```python
from build123d import *

# Parameters (mm, degrees)
F0_W     = 10
F0_H     = 20
F0_R     = 2.65
F1_DEPTH = 2.2
F2_R     = 0.5


with BuildPart() as f1:
    # F0 (on Top) → F1 (new body)
    with BuildSketch(Plane.XY):
        Rectangle(F0_W, F0_H)
        Circle(F0_R, mode=Mode.SUBTRACT)
    extrude(amount=F1_DEPTH)

    # F2
    f2_edges = [f1.edges().sort_by_distance(p)[0] for p in [
        (-2.65, 0, 2.2),
        (5, 0, 2.2),
        (0, 10, 2.2),
        (0, -10, 2.2),
        (-5, 0, 2.2),
    ]]
    fillet(f2_edges, radius=F2_R)


solid = f1.part
```
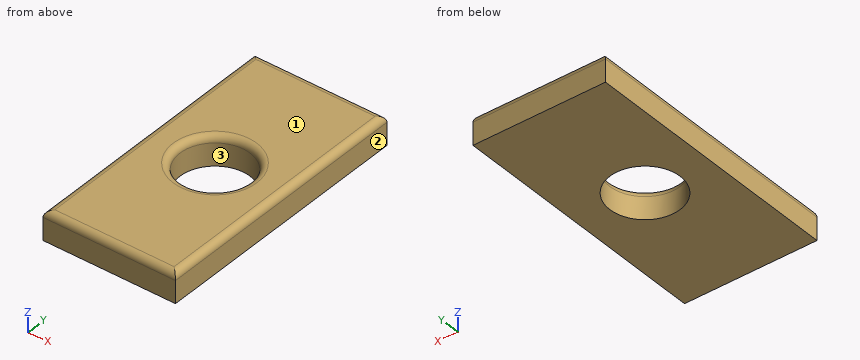
For this review, take the finished solid that the model builds, in its own axes (mm). Face numbers are marked on the shaded views. Coordinates: 2 decimals unless noted, no trailing zeros. Write each loop counter-clockwise with the first axis right and the second up, starting at its lowest first coordinate (ties: lowest second). Pieces come first, ordered by that corner, then holes. Notation, with made-up numbers: (3, -25.75) - (20, -25.75) arc R9 ccw to (20, -21.75) - close; hole circle Ø5 at (-26.75, -40). An arc over 180 degrees is marked (long way). Answer in a Markdown table with one row per item. Add a question column.
Q1. For probe 1 along Y at (x, z) = (0, 0.65); probe 2 along X at (y, z) = (1.5, 1.9); probe 3 along Y at (x, z) = (-2, 0.1), list the stretches that pass through material, from the lowest coordinate up.
Q2. We need section B-B, the plane y = 0. State the section outline as (x, z) points, and give its area (3 significant figures).
Q3. We need section C-C, the plane z = 1.5. State the section outline as (x, y) points, and give its area (3 significant figures).
Q4. Draft analysis for pull direction X (two halves, no side actions). For the marked faces 1, 2 and 3, state which applies: +X half, -X half, draft (parallel to the pull), parting line (faces both ways), or undercut.
Q5. For P1, Ø6, axis at x = 0, y = 0, coming from the +Z side, flat-tipped, find the tip position at first contact; note if it passes through.
Q6. We need section A-A, the plane x = 0. State the section outline as (y, z) points, and give its area (3 significant figures).
Answer list:
| question | item | result |
|---|---|---|
| 1 | probe 1 | y = -10 to -2.65, 2.65 to 10 |
| 1 | probe 2 | x = -4.96 to -2.24, 2.24 to 4.96 |
| 1 | probe 3 | y = -10 to -1.74, 1.74 to 10 |
| 2 | outline | (-5, 0) - (-2.65, 0) - (-2.65, 1.7) arc R0.5 ccw to (-3.15, 2.2) - (-4.5, 2.2) arc R0.5 ccw to (-5, 1.7) - close; (2.65, 0) - (5, 0) - (5, 1.7) arc R0.5 ccw to (4.5, 2.2) - (3.15, 2.2) arc R0.5 ccw to (2.65, 1.7) - close |
| 2 | area | 10.1 mm2 |
| 3 | outline | (-5, -10) - (5, -10) - (5, 10) - (-5, 10) - close; hole circle Ø5.3 at (0, 0) |
| 3 | area | 178 mm2 |
| 4 | face 1 | draft |
| 4 | face 2 | +X half |
| 4 | face 3 | undercut |
| 5 | P1 | stops at z = 2.18 |
| 6 | outline | (-10, 0) - (-2.65, 0) - (-2.65, 1.7) arc R0.5 ccw to (-3.15, 2.2) - (-9.5, 2.2) arc R0.5 ccw to (-10, 1.7) - close; (2.65, 0) - (10, 0) - (10, 1.7) arc R0.5 ccw to (9.5, 2.2) - (3.15, 2.2) arc R0.5 ccw to (2.65, 1.7) - close |
| 6 | area | 32.1 mm2 |
